The model under review builds one solid part; all positions refer to its coordinate system, in mm. Coordinates: 2 decimals unless noted, no trailing zeros. Loops run counter-clockwise (first coordinate to the right, second up) from the corner with the lowest first, then second, coordinate; pieces in that order, holes last. Notation, with made-up numbers: M 30.25,-29 L 63.25,-29 A28 cw 63.25,-3 Z; hole C -10.75,33.25 d5. An arc over 180 degrees is marked long. One line per item, written item: value.
```python
from build123d import *

# Parameters (mm, degrees)
F0_W     = 43.5587465763
F0_H     = 42.1372503042
F0_R     = 14.2222248189
F1_DEPTH = 25.4
F2_SIZE  = 2.54
F3_R     = 0.762
F4_R     = 5.08


with BuildPart() as f1:
    # F0 (on Top) → F1 (new body)
    with BuildSketch(Plane.XY):
        with Locations((21.7793732882, 21.0686251521)):
            Rectangle(F0_W, F0_H)
        with Locations((18.9871452749, 21.6270685196)):
            Circle(F0_R, mode=Mode.SUBTRACT)
    extrude(amount=F1_DEPTH)

    # F2
    f2_edges = [f1.edges().sort_by_distance(p)[0] for p in [
        (4.76492, 21.627069, 25.4),
    ]]
    chamfer(f2_edges, length=F2_SIZE)

    # F3
    f3_edges = [f1.edges().sort_by_distance(p)[0] for p in [
        (2.22492, 21.627069, 25.4),
    ]]
    fillet(f3_edges, radius=F3_R)

    # F4
    f4_edges = [f1.edges().sort_by_distance(p)[0] for p in [
        (4.76492, 21.627069, 22.86),
    ]]
    fillet(f4_edges, radius=F4_R)


solid = f1.part
```
(1) Insertion check: pin 1 Ø5 at (x, y) = (5.5, 23) entering from +Z; pin 2 Ø8 at (x, y) = (25, 18.5) entering from -Z. Each pin has a flat end and moves straight along its axis. Give the tip position at first contact, or say it passes through.
Checks:
pin 1: z = 24.69
pin 2: through
(2) Draft analysis for pull direction X (two halves, no side actions). For faces 1 (the face through (43.559, 21, 13)), 2 (the face through (17.14, 35.73, 10.23)), 3 (the face through (0, 21, 13)), 4 (the face through (36, 17, 25.4)), state which applies: pulls with the +X half, pulls with the -X half, needs draft (parallel to the pull), parting line crosses it, or undercut.
Checks:
face 1: pulls with the +X half
face 2: undercut
face 3: pulls with the -X half
face 4: needs draft
(3) Add section A-A on z = 6.25. State the section outline as (x, y) points.
Checks:
outline: M 0,0 L 43.56,0 L 43.56,42.14 L 0,42.14 Z; hole C 18.99,21.63 d28.44
(4) To check wall thickness, follow L1, parallel to Y at x = 24.5, z = 17.25; L2, parallel to X at y = 31, z = 1.5; L3, parallel to Y at x = 12, z = 17. State the ranges of each line that lie inside material, in increasing order. Write a range as [from, to].
Checks:
L1: [0, 8.52], [34.74, 42.14]
L2: [0, 8.29], [29.68, 43.56]
L3: [0, 9.24], [34.01, 42.14]
